Model file for the job. Use its own axes, mm. Face numbers are marked on the shaded views. A direction names the side the tool comes from. Round coordinates to 2 decimals unless told otherwise and drop trailing zeros. Loops run counter-clockwise (first coordinate to the right, second up) from the corner with the lowest first, then second, coordinate; pieces in that order, holes last. Notation, with made-up numbers: M -28.75,82.5 L -3.75,82.5 A7 cw -3.75,89.5 Z; hole C 38,70.5 d2. An arc over 180 degrees is marked long. Use a Markdown table: item, result. Add a question column.
Item 1: Tool access for the marked faces 4, 5, 6, 7 and 8: list every direction of +Z, -Z, +X, -X, +Y, -Y with a clear straight run to the whole face (end or side of a thin tool).
Item 2: Pin check, flat tips, straight feed: P1, Ø9.5, axis at x = 6.5, y = 19, coming from the +Z side; P2, Ø1, axis at y = 10, z = 9.5, coming from the +X side; P3, Ø4, axis at x = 7, z = 17, coming from the +Y side; P4, Ø5, axis at x = 6.35, z = -6.35, coming from the +Y side. Stop position of each tip, or through.
Item 3: Saw through at C-C on x = 6.75. Give the number of separate pieces and of enclosed holes in the cut face, then the cut area to 3 significant figures.
Item 4: Wall check: L1, parallel to Z at x = 6.35, y = 2.8 (3 decimals); L2, parallel to X at y = 3.9, z = -6.35 (3 decimals); L3, parallel to Z at x = 7.5, y = 1.75. Give the ranges that are in metal, low to high. Write a range as from..to.
Item 5: Saw through at D-D on z = 23. Write the cut outline in (x, y), then the cut area to 3 significant figures.
Item 6: Saw through at A-A on z = 19.05. Write the cut outline in (x, y) (3 decimals).
Item 7: Saw through at B-B on x = 1.5. Write the cut outline in (y, z).
Item 8: Two-plate mould, pull along X, no slides. Class the marked faces 1, 2 and 3: +X half, -X half, draft (parallel to the pull), parting line (faces both ways), or undercut.
```python
from build123d import *

# Parameters (mm, degrees)
BOSS_EXTRUDE3_DEPTH = 12.7
SKETCH8_R           = 2
CUT_EXTRUDE5_DEPTH  = 12.7
CUT_EXTRUDE7_DEPTH  = 12.7
SKETCH10_W          = 12.7
SKETCH10_H          = 5.08
BOSS_EXTRUDE4_DEPTH = 12.7
SKETCH11_R          = 3.175
CUT_EXTRUDE8_DEPTH  = 12.7
SKETCH13_R          = 3
SKETCH13_R_2        = 2
BOSS_EXTRUDE5_DEPTH = 1.27


with BuildPart() as part:
    # Sketch7 → Boss-Extrude3 (new body)
    with BuildSketch(Plane.XY):
        Polygon((0, 12.027702426), (12.192, 25.102021739), (24.892, 25.102021739), (12.7, 12.027702426), (12.7, 0), (0, 0), align=None)
    extrude(amount=BOSS_EXTRUDE3_DEPTH)

    # Sketch8 → Cut-Extrude5 (cut)
    with BuildSketch(Plane(origin=(-5.999201774, 5.594346159, 0), x_dir=(0, 0, 1), z_dir=(-0.731353702, 0.68199836, 0))):
        with Locations((6.35, 17.734942607)):
            Circle(SKETCH8_R)
    extrude(amount=-CUT_EXTRUDE5_DEPTH, mode=Mode.SUBTRACT)

    # Sketch9 → Cut-Extrude7 (cut)
    with BuildSketch(Plane.XY.offset(12.7)):
        Polygon((12.192, 25.102021739), (18.984953608, 18.76749002), (24.892, 25.102021739), align=None)
    extrude(amount=-CUT_EXTRUDE7_DEPTH, mode=Mode.SUBTRACT)

    # Sketch10 → Boss-Extrude4 (add)
    with BuildSketch(Plane.XY.offset(12.7)):
        with Locations((6.35, 2.54)):
            Rectangle(SKETCH10_W, SKETCH10_H)
    boss_extrude4 = extrude(amount=BOSS_EXTRUDE4_DEPTH)

    # Sketch11 → Cut-Extrude8 (cut)
    with BuildSketch(Plane(origin=(0, 5.08, 0), x_dir=(1, 0, 0), z_dir=(0, 1, 0))):
        with Locations((6.35, -19.05)):
            Circle(SKETCH11_R)
    cut_extrude8 = extrude(amount=-CUT_EXTRUDE8_DEPTH, mode=Mode.SUBTRACT)

    # Mirror2: Boss-Extrude4, Cut-Extrude8 across plane
    add(boss_extrude4.mirror(Plane.XY.offset(6.35)))
    add(cut_extrude8.mirror(Plane.XY.offset(6.35)), mode=Mode.SUBTRACT)

    # Sketch13 → Boss-Extrude5 (add)
    with BuildSketch(Plane(origin=(-5.999201774, 5.594346159, 0), x_dir=(0, 0, 1), z_dir=(-0.731353702, 0.68199836, 0))):
        with Locations((6.35, 17.734942607)):
            Circle(SKETCH13_R)
        with Locations((6.35, 17.734942607)):
            Circle(SKETCH13_R_2, mode=Mode.SUBTRACT)
    extrude(amount=BOSS_EXTRUDE5_DEPTH)


solid = part.part
```
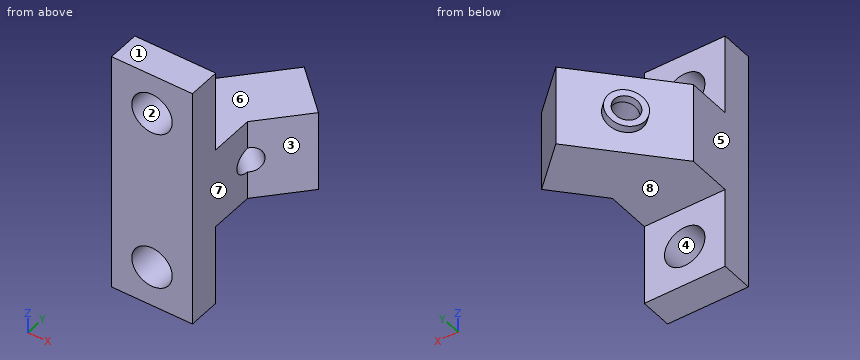
Entries:
| question | item | result |
|---|---|---|
| 1 | face 4 | +Y, -Y |
| 1 | face 5 | +Z, -Z, -X, +Y, -Y |
| 1 | face 6 | +Z, +X, -X, +Y |
| 1 | face 7 | +Z, -Z, +X, -Y |
| 1 | face 8 | -Z, +X, -X, +Y |
| 2 | P1 | z = 12.7 |
| 2 | P2 | x = 12.7 |
| 2 | P3 | y = 5.08 |
| 2 | P4 | through |
| 3 | separate pieces | 3 |
| 3 | enclosed holes | 1 |
| 3 | area | 302 mm2 |
| 4 | L1 | -12.7..-9.525, -3.175..15.875, 22.225..25.4 |
| 4 | L2 | 0..3.175, 9.525..12.7 |
| 4 | L3 | -12.7..-9.31, -3.39..16.09, 22.01..25.4 |
| 5 | outline | M 0,0 L 12.7,0 L 12.7,5.08 L 0,5.08 Z |
| 5 | area | 64.5 mm2 |
| 6 | outline | M 0,0 L 3.175,0 L 3.175,5.08 L 0,5.08 Z; M 9.525,0 L 12.7,0 L 12.7,5.08 L 9.525,5.08 Z |
| 7 | outline | M 0,-12.7 L 5.08,-12.7 L 5.08,0 L 13.64,0 L 13.64,12.7 L 5.08,12.7 L 5.08,25.4 L 0,25.4 Z |
| 8 | face 1 | draft |
| 8 | face 2 | undercut |
| 8 | face 3 | +X half |
